Part model, mm, in its own coordinate system. A direction names the side the tool comes from. Round coordinates to 2 decimals unless told otherwise and drop trailing zeros. Write each loop counter-clockwise with the first axis right and the second up, starting at its lowest first coordinate (ties: lowest second). Pieces come first, ordered by that corner, then holes.
1) Saw through at A-A on x = 61.5. Write the cut outline in (y, z), and give its area (3 significant figures).
2) Which spindle directions (+Z, -Z, +X, -X, +Y, -Y) get a long thin tool onto all of the face, cutting with end or side? Do faces 1 (the flat face through (74, 15, -15)), 2 (the flat face through (18, 10, -3)). Say none if no direction does.
3) Pull direction Z, two halves, no side cores. Call faces 3 (the flat face through (39, 7, 0)), 4 (the flat face through (61, 10, -27)), 5 (the flat face through (39, 0, -15)): +Z half, -Z half, draft (parallel to the pull), parting line (faces both ways), or undercut.
4) Flat gauge pin, fed straight in: pin 1 (2 mm diameter, centred on x = 56, z = -18.5, fed in from +Y). Where does the tip first touch, or does it go through?
5) Drill centre lines: L1, parallel to X at y = 9, z = -3.75; L2, parallel to X at y = 14.75, z = -16; L3, parallel to Y at x = 18.5, z = -26.5. Where is each one in solid material? Low to high.
6) Saw through at B-B on z = -18.5. Write the cut outline in (x, y).
```python
from build123d import *

# Parameters (mm, degrees)
SKETCH1_W               = 80
SKETCH1_H               = 30
BOSS_EXTRUDE1_DEPTH     = 15
SKETCH2_R               = 7.5
CUT_EXTRUDE1_DEPTH      = 87.746757864
SKETCH3_W               = 15
SKETCH3_H               = 3
BOSS_EXTRUDE2_DEPTH     = 10
CUT_EXTRUDE2_DEPTH      = 87.746757864
CUT_EXTRUDE2_DEPTH_BACK = 87.746757864
SKETCH4_R               = 4.5


with BuildPart() as part:
    # Sketch1 → Boss-Extrude1 (new body)
    with BuildSketch(Plane(origin=(0, 0, 0), x_dir=(1, 0, 0), z_dir=(0, 1, 0))):
        with Locations((40, 15)):
            Rectangle(SKETCH1_W, SKETCH1_H)
    extrude(amount=BOSS_EXTRUDE1_DEPTH)

    # Sketch2 → Cut-Extrude1 (cut, through all)
    with BuildSketch(Plane.XY):
        with Locations((18.5, 15)):
            Circle(SKETCH2_R)
        with Locations((61.5, 15)):
            Circle(SKETCH2_R)
    extrude(amount=-CUT_EXTRUDE1_DEPTH, mode=Mode.SUBTRACT)

    # Sketch3 → Boss-Extrude2 (add)
    with BuildSketch(Plane(origin=(0, 15, 0), x_dir=(1, 0, 0), z_dir=(0, 1, 0))):
        with Locations((18.5, 1.5)):
            Rectangle(SKETCH3_W, SKETCH3_H)
        with Locations((61.5, 28.5)):
            Rectangle(SKETCH3_W, SKETCH3_H)
        with Locations((61.5, 1.5)):
            Rectangle(SKETCH3_W, SKETCH3_H)
        with Locations((18.5, 28.5)):
            Rectangle(SKETCH3_W, SKETCH3_H)
    extrude(amount=-BOSS_EXTRUDE2_DEPTH)

    # Sketch4 → Cut-Extrude2 (cut, two sides: drawn at the far end of the back side and taken through both)
    with BuildSketch(Plane.XY.offset(-CUT_EXTRUDE2_DEPTH_BACK)):
        with Locations((18.5, 15)):
            Circle(SKETCH4_R)
        with Locations((61.5, 15)):
            Circle(SKETCH4_R)
    extrude(amount=CUT_EXTRUDE2_DEPTH + CUT_EXTRUDE2_DEPTH_BACK, mode=Mode.SUBTRACT)


solid = part.part
```
Completed:
1. outline: (0, -30) - (10.5, -30) - (10.5, -27) - (7.5, -27) - (7.5, -3) - (10.5, -3) - (10.5, 0) - (0, 0) - close
1. area: 243 mm2
2. face 1: +Z, -Z, +X, -X, +Y
2. face 2: +Y
3. face 3: +Z half
3. face 4: undercut
3. face 5: draft
4. pin 1: stops at y = 11.26
5. L1: x = 0 to 14, 23 to 57, 66 to 80
5. L2: x = 0 to 11, 26 to 54, 69 to 80
5. L3: y = 0 to 7.5
6. outline: (0, 0) - (80, 0) - (80, 15) - (69, 15) arc R7.5 cw to (54, 15) - (26, 15) arc R7.5 cw to (11, 15) - (0, 15) - close
